For this review, take the finished solid that the model builds, in its own axes (mm). Round coordinates to 2 decimals unless told otherwise and drop trailing zeros. Order: outer loops, then holes, each group sorted by start corner. A loop starts at its lowest first (then second) coordinate and runs counter-clockwise, first axis right, second up. Notation, with made-up numbers: (-13, -20.5) -> (32, -20.5) arc R17 ccw to (32, -0.5) -> close; hole circle Ø3 at (-39, -33.5). An arc over 180 degrees is marked (long way). Put each result on its own line as item: value. Start each with the question number.
```python
from build123d import *

# Parameters (mm, degrees)
SKETCH_1_W         = 30
SKETCH_1_H         = 6
EXTRUDE_1_DEPTH    = 6
HOLE_WIZARD_M3_1_D = 2.5
HOLE_WIZARD_M3_2_D = 2.5
HOLE_WIZARD_M3_3_D = 2.5


with BuildPart() as part:
    # 草图1 → 凸台-拉伸1 (new body)
    with BuildSketch(Plane(origin=(0, 0, 0), x_dir=(0, 0, -1), z_dir=(1, 0, 0))):
        with Locations((15, 3)):
            Rectangle(SKETCH_1_W, SKETCH_1_H)
    extrude(amount=EXTRUDE_1_DEPTH)

    # M3 螺纹孔1 (through all)
    with Locations(Plane.XY):
        with Locations((3, 3)):
            Hole(HOLE_WIZARD_M3_1_D / 2)

    # M3 螺纹孔2 (through all)
    with Locations(Plane(origin=(0, 6, 0), x_dir=(1, 0, 0), z_dir=(0, 1, 0))):
        with Locations((3, 12.5), (3, 22.5)):
            Hole(HOLE_WIZARD_M3_2_D / 2)

    # M3 螺纹孔3 (through all)
    with Locations(Plane(origin=(6, 0, 0), x_dir=(0, 0, -1), z_dir=(1, 0, 0))):
        with Locations((17.5, 3), (7.5, 3)):
            Hole(HOLE_WIZARD_M3_3_D / 2)


solid = part.part
```
Item 1: Mouldability with a two-part tool opening along Y and no side actions: class faces 1 (the face through (2.423, 4.812, -11.391)), 2 (the face through (1.146, 4.054, -6.828)), 3 (the face through (3, 0, -15)) as +Y half, -Y half, draft (parallel to the pull), parting line (faces both ways), or undercut.
Item 2: Consider section A-A, the plane z = -2.5. Write out the cut boundary in (x, y).
Item 3: Consider section D-D, the plane z = -12. Write out the cut boundary in (x, y), plus the area to 3 significant figures.
Item 4: For L1, parallel to Z at x = 1.35, y = 3; L2, parallel to X at y = 3, z = -21.1; L3, parallel to Z at x = 5.6, y = 3.5, list the stretches that pass through material, from the lowest coordinate up.
Item 5: Insertion check: pin 1 Ø2 at (x, y) = (3, 3) entering from -Z; pin 2 Ø2 at (x, y) = (2.5, 3.5) entering from +Z. Each pin has a flat end and moves straight along its axis. Give the tip position at first contact, or say it passes through.
Item 6: Consider section B-B, the plane x = 4.55. Write out the cut boundary in (y, z).
Item 7: Consider section C-C, the plane y = 0.7. Write out the cut boundary in (x, z), plus the area to 3 significant figures.
Evaluation:
1. face 1: draft
1. face 2: undercut
1. face 3: -Y half
2. outline: (0, 0) -> (6, 0) -> (6, 6) -> (0, 6) -> close; hole circle Ø2.5 at (3, 3)
3. outline: (0, 0) -> (1.85, 0) -> (1.85, 2.5) arc R1.25 cw to (1.85, 3.5) -> (1.85, 6) -> (0, 6) -> close; (4.15, 0) -> (6, 0) -> (6, 6) -> (4.15, 6) -> (4.15, 3.5) arc R1.25 cw to (4.15, 2.5) -> close
3. area: 22.1 mm^2
4. L1: z = -30 to -18.75, -16.25 to -8.75, -6.25 to 0
4. L2: x = 0 to 1.75, 4.25 to 6
4. L3: z = -30 to -18.65, -16.35 to -8.65, -6.35 to 0
5. pin 1: passes through
5. pin 2: stops at z = 0
6. outline: (0, -30) -> (6, -30) -> (6, 0) -> (0, 0) -> close; hole circle Ø2.5 at (3, -17.5); hole circle Ø2.5 at (3, -7.5)
7. outline: (0, -30) -> (6, -30) -> (6, 0) -> (0, 0) -> close; hole circle Ø2.5 at (3, -22.5); hole circle Ø2.5 at (3, -12.5)
7. area: 170 mm^2
